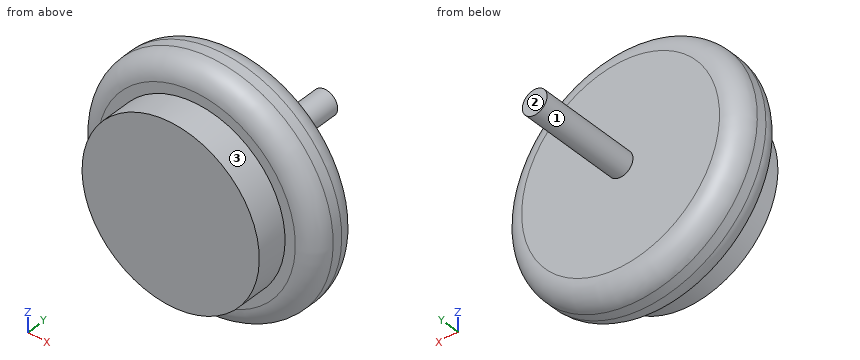
```python
from build123d import *

# Parameters (mm, degrees)
SKETCH1_R           = 58
BOSS_EXTRUDE1_DEPTH = 25
SKETCH2_R           = 43
BOSS_EXTRUDE2_DEPTH = 15
FILLET1_R           = 10
BOSS_EXTRUDE3_START = 25
SKETCH3_R           = 6
BOSS_EXTRUDE3_DEPTH = 50


with BuildPart() as part:
    # Sketch1 → Boss-Extrude1 (new body)
    with BuildSketch(Plane(origin=(0, 0, 0), x_dir=(1, 0, 0), z_dir=(0, 1, 0))):
        with Locations(Location((0, 0, 0), (0, 0, 270))):
            Circle(SKETCH1_R)
    extrude(amount=BOSS_EXTRUDE1_DEPTH)

    # Sketch2 → Boss-Extrude2 (add)
    with BuildSketch(Plane(origin=(0, 0, 0), x_dir=(1, 0, 0), z_dir=(0, 1, 0))):
        with Locations(Location((0, 0, 0), (0, 0, 270))):
            Circle(SKETCH2_R)
    extrude(amount=-BOSS_EXTRUDE2_DEPTH)

    # Fillet1
    fillet1_edges = [part.edges().sort_by_distance(p)[0] for p in [
        (0, 0, -58),
        (0, 25, -58),
    ]]
    fillet(fillet1_edges, radius=FILLET1_R)

    # Sketch3 → Boss-Extrude3 (add)
    with BuildSketch(Plane(origin=(0, 0, 0), x_dir=(1, 0, 0), z_dir=(0, 1, 0)).offset(BOSS_EXTRUDE3_START)):
        with Locations(Location((0, 0, 0), (0, 0, 270))):
            Circle(SKETCH3_R)
    extrude(amount=BOSS_EXTRUDE3_DEPTH)


solid = part.part
```
Can you work these out from the model? Positions are in its coordinate system, mm. Face numbers are marked on the shaded views. A direction names the side the tool comes from. Give positions to 0.01 mm unless a question says otherwise; leave off trailing zeros. Write each loop counter-clockwise with the first axis right and the second up, starting at its lowest first coordinate (ties: lowest second). Pieces come first, ordered by that corner, then holes. Notation, with made-up numbers: (-35, 75) - (21, 75) arc R27 cw to (21, 91) - close; hole circle Ø3 at (63, 78). An arc over 180 degrees is marked (long way). Write item = value, one per line. Start each with the question number.
1. Imagine slicing it at B-B (x = 0). Please give me the cut outline in (y, z).
2. Please list where these lines run through material, in increasing order: line 1 (Y direction, x = -28, z = 5.5); line 2 (Z direction, x = -3, y = 70); line 3 (X direction, y = 5, z = -5).
3. For pin 1 (6 mm diameter, centred on x = -23.5, y = 3, fed in from +Z); pin 2 (3 mm diameter, centred on y = -3.5, z = 35, fed in from -X); pin 3 (1.5 mm diameter, centred on y = 6.5, z = 14.5, fed in from -X), each with a flat end and sliding along its axis, tell me the tip position at first contact or that it passes through.
4. On a 3-axis mill with a long thin cutter (end or side, diameter ignored), from which of +Z, -Z, +X, -X, +Y, -Y can I reach the whole of each face in a straight line? I mean the marked faces 1, 2 and 3. Say none if no direction works.
5. Imagine slicing it at D-D (y = 6.5). Please give me the cut outline in (x, z) (1 decimal), and give its area (3 significant figures).
6. Imagine slicing it at C-C (y = 30). Please give me the cut outline in (x, z), and give its area (3 significant figures).
7. Imagine slicing it at A-A (z = 0). Please give me the cut outline in (x, y), and give its area (3 significant figures).
Worked answers:
q1.outline = (-15, -43) - (0, -43) - (0, -48) arc R10 ccw to (10, -58) - (15, -58) arc R10 ccw to (25, -48) - (25, -6) - (75, -6) - (75, 6) - (25, 6) - (25, 48) arc R10 ccw to (15, 58) - (10, 58) arc R10 ccw to (0, 48) - (0, 43) - (-15, 43) - close
q2.line_1 = -15 to 25
q2.line_2 = -5.2 to 5.2
q2.line_3 = -56.44 to 56.44
q3.pin_1 = 52.58
q3.pin_2 = -26.96
q3.pin_3 = -55.83
q4.face_1 = +Y
q4.face_2 = +Z, -Z, +X, -X, +Y
q4.face_3 = -Y
q5.outline = circle Ø114.7 at (0, 0)
q5.area = 10,300 mm2
q6.outline = circle Ø12 at (0, 0)
q6.area = 113 mm2
q7.outline = (-58, 10) arc R10 ccw to (-48, 0) - (-43, 0) - (-43, -15) - (43, -15) - (43, 0) - (48, 0) arc R10 ccw to (58, 10) - (58, 15) arc R10 ccw to (48, 25) - (6, 25) - (6, 75) - (-6, 75) - (-6, 25) - (-48, 25) arc R10 ccw to (-58, 15) - close
q7.area = 4,700 mm2
